For this review, take the finished solid that the model builds, in its own axes (mm). Coordinates: 2 decimals unless noted, no trailing zeros. Loops run counter-clockwise (first coordinate to the right, second up) from the corner with the lowest first, then second, coordinate; pieces in that order, holes last. Notation, with made-up numbers: M 29,63 L 64,63 A14 cw 64,82 Z; hole C 63,26.5 d3. An arc over 180 degrees is marked long. Write item = value, one per line.
from build123d import *

# Parameters (mm, degrees)
SKETCH1_R           = 6.5
BOSS_EXTRUDE2_DEPTH = 15


with BuildPart() as part:
    # Sketch1 → Boss-Extrude2 (new body)
    with BuildSketch(Plane(origin=(0, 0, 0), x_dir=(0, 1, 0), z_dir=(0, 0, 1))):
        Polygon((0, 60), (0, 0), (60, 0), (60, 15), (25, 60), align=None)
        with Locations(Location((25, 40, 0), (0, 0, 270))):
            Circle(SKETCH1_R, mode=Mode.SUBTRACT)
    extrude(amount=-BOSS_EXTRUDE2_DEPTH)


solid = part.part
Q1. For line 1 along Y through (x, z) = (-41.5, -8.5); line 2 along Y through (x, z) = (-40, -6.25); line 3 along X through (y, z) = (21.5, -12), list the stretches that pass through material, from the lowest coordinate up.
Solved:
line_1 = 0 to 18.68, 31.32 to 39.39
line_2 = 0 to 18.5, 31.5 to 40.56
line_3 = -60 to -45.48, -34.52 to 0
Q2. Add section B-B (x = -49). Write out the cut boundary in (y, z).
Solved:
outline = M 0,-15 L 33.56,-15 L 33.56,0 L 0,0 Z
Q3. Draft analysis for pull direction Y (two halves, no side actions). For faces 1 (the face through (-46.494, 25.286, -7.395)), 2 (the face through (-7, 60, -7)), 3 (the face through (-30, 0, -7)), 4 (the face through (0, 30, -7)), state which applies: +Y half, -Y half, draft (parallel to the pull), parting line (faces both ways), or undercut.
Solved:
face_1 = undercut
face_2 = +Y half
face_3 = -Y half
face_4 = draft
Q4. For pin 1 Ø15 at (x, y) = (-40, 25) entering from +Z; pin 2 Ø2 at (x, y) = (-41.5, 43) entering from -Z, all flat-tipped, find the tip position at first contact; note any pin that passes through.
Solved:
pin_1 = 0
pin_2 = through
Q5. Add section A-A (x = -40). Write out the cut boundary in (y, z), and give its area (3 significant figures).
Solved:
outline = M 0,-15 L 18.5,-15 L 18.5,0 L 0,0 Z; M 31.5,-15 L 40.56,-15 L 40.56,0 L 31.5,0 Z
area = 413 mm²
Q6. Add section C-C (y = 33). Write out the cut boundary in (x, z).
Solved:
outline = M -49.71,-15 L 0,-15 L 0,0 L -49.71,0 Z
